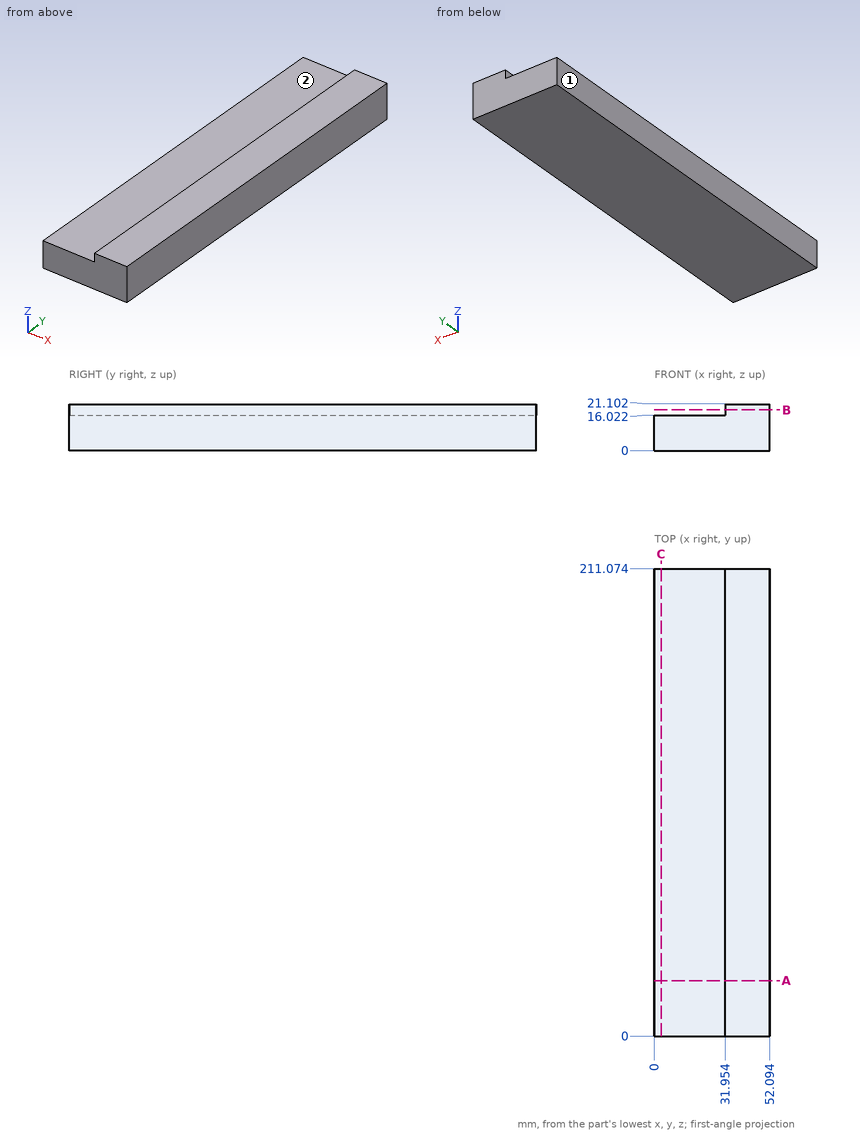
Here's the drawing with two shaded views (mm, measured from the low corner). I have some questions. A direction names the side the tool comes from. Round coordinates to 2 decimals unless told otherwise and drop trailing zeros. Loops run counter-clockwise (first coordinate to the right, second up) from the corner with the lowest first, then second, coordinate; pieces in that order, holes last.
Item 1: Suppose I cut it at A-A, the plane y = 25. Write out the boundary of the cut face in (x, z) (1 decimal), then the cut area to 3 significant figures.
Item 2: Will these pins go through, and if not, where does the flat tip stop? pin 1 Ø9.5 at (x, y) = (14.5, 116) entering from +Z; pin 2 Ø1.5 at (y, z) = (144.5, 19.5) entering from -X.
Item 3: Suppose I cut it at B-B, the plane z = 18.5. Write out the boundary of the cut face in (x, y) (1 decimal).
Item 4: Which directions (+Z, -Z, +X, -X, +Y, -Y) give clear straight access to the entire face, cutting with the end or side of a thin tool? Please do the marked faces 1 and 2.
Item 5: Please list where this line runs through material, in increasing order: L1, parallel to Z at x = 20.5, y = 181.
Item 6: Suppose I cut it at C-C, the plane x = 3. Write out the boundary of the cut face in (y, z), then the cut area to 3 significant figures.
Reported:
1. outline: (0, 0) - (52.1, 0) - (52.1, 21.1) - (32, 21.1) - (32, 16) - (0, 16) - close
1. area: 937 mm2
2. pin 1: stops at z = 16.02
2. pin 2: stops at x = 31.95
3. outline: (32, 0) - (52.1, 0) - (52.1, 211.1) - (32, 211.1) - close
4. face 1: +Z, -Z, -X, +Y, -Y
4. face 2: +Z, -X, +Y, -Y
5. L1: z = 0 to 16.02
6. outline: (0, 0) - (211.07, 0) - (211.07, 16.02) - (0, 16.02) - close
6. area: 3,380 mm2
